from build123d import *

# Parameters (mm, degrees)
BOSS_EXTRU_1_DEPTH                              = 8
CHAMBRAGE_POUR_VIS_T_TE_CYLINDRIQUE_D           = 2.5
CHAMBRAGE_POUR_VIS_T_TE_CYLINDRIQUE_CBORE_D     = 4.5
CHAMBRAGE_POUR_VIS_T_TE_CYLINDRIQUE_CBORE_DEPTH = 6.5
CONG_1_R                                        = 0.5
ESQUISSE6_R                                     = 1.6
ENL_V_MAT_EXTRU_1_DEPTH                         = 18.49285573
ESQUISSE7_W                                     = 6
ESQUISSE7_H                                     = 2.25
ENL_V_MAT_EXTRU_2_DEPTH                         = 18.492855685
ESQUISSE8_R                                     = 5.5
ENL_V_MAT_EXTRU_3_DEPTH                         = 3


with BuildPart() as part:
    # Esquisse1 → Boss.-Extru.1 (new body)
    with BuildSketch(Plane(origin=(0, 0, 0), x_dir=(1, 0, 0), z_dir=(0, 1, 0))):
        with BuildLine():
            Line((4.582575695, 10), (-4.582575695, 10))
            ThreePointArc((-4.582575695, 10), (0, -11), (4.582575695, 10))
        make_face()
        with BuildLine():
            Line((-3.2, 0), (-3.2, 2.9))
            Line((-3.2, 2.9), (3.2, 2.9))
            Line((3.2, 2.9), (3.2, 0))
            ThreePointArc((3.2, 0), (0, -3.2), (-3.2, 0))
        make_face(mode=Mode.SUBTRACT)
    extrude(amount=BOSS_EXTRU_1_DEPTH)

    # Chambrage pour vis à tête cylindrique à 6 pans creux (ou vis CHC) M21 (through all)
    with Locations(Plane(origin=(0, 8, 0), x_dir=(1, 0, 0), z_dir=(0, 1, 0))):
        with Locations((5.656854249, 5.656854249), (5.656854249, -5.656854249), (-5.656854249, -5.656854249), (-5.656854249, 5.656854249), (0, 0)):
            CounterBoreHole(CHAMBRAGE_POUR_VIS_T_TE_CYLINDRIQUE_D / 2, CHAMBRAGE_POUR_VIS_T_TE_CYLINDRIQUE_CBORE_D / 2, CHAMBRAGE_POUR_VIS_T_TE_CYLINDRIQUE_CBORE_DEPTH)

    # Congé1
    cong_1_edges = [part.edges().sort_by_distance(p)[0] for p in [
        (0, 8, 3.2),
        (3.2, 8, -1.45),
        (0, 8, -2.9),
        (-3.2, 8, -1.45),
    ]]
    fillet(cong_1_edges, radius=CONG_1_R)

    # Esquisse6 → Enlèv. mat.-Extru.1 (cut, through all)
    with BuildSketch(Plane.XY):
        with Locations((0, 5.5)):
            Circle(ESQUISSE6_R)
    extrude(amount=-ENL_V_MAT_EXTRU_1_DEPTH, mode=Mode.SUBTRACT)

    # Esquisse7 → Enlèv. mat.-Extru.2 (cut, through all)
    with BuildSketch(Plane(origin=(0, 8, 0), x_dir=(1, 0, 0), z_dir=(0, 1, 0))):
        with Locations((0, 5.025)):
            Rectangle(ESQUISSE7_W, ESQUISSE7_H)
    extrude(amount=-ENL_V_MAT_EXTRU_2_DEPTH, mode=Mode.SUBTRACT)

    # Esquisse8 → Enlèv. mat.-Extru.3 (cut)
    with BuildSketch(Plane(origin=(0, 0, 0), x_dir=(-1, 0, 0), z_dir=(0, -1, 0))):
        Circle(ESQUISSE8_R)
    extrude(amount=-ENL_V_MAT_EXTRU_3_DEPTH, mode=Mode.SUBTRACT)


solid = part.part
Model file for the job. Use its own axes, mm. A direction names the side the tool comes from. Give positions to 0.01 mm unless a question says otherwise; leave off trailing zeros. Write each loop counter-clockwise with the first axis right and the second up, starting at its lowest first coordinate (ties: lowest second). Pieces come first, ordered by that corner, then holes. Notation, with made-up numbers: (82, -0.75) - (98, -0.75) arc R21 ccw to (98, 20.25) - close; hole circle Ø9 at (81.5, 7.25). An arc over 180 degrees is marked (long way). Answer as CSV lines item,"result".
1. Band-saw the part on D-D (y = 5.5). Write the cut outline in (x, z), and give its area (3 significant figures).
Responses:
outline,"(-4.58, -10) - (-1.6, -10) - (-1.6, -6.15) - (-3, -6.15) - (-3, -3.9) - (-1.6, -3.9) - (-1.6, -2.9) - (-3.2, -2.9) - (-3.2, 0) arc R3.2 cw to (3.2, 0) - (3.2, -2.9) - (1.6, -2.9) - (1.6, -3.9) - (3, -3.9) - (3, -6.15) - (1.6, -6.15) - (1.6, -10) - (4.58, -10) arc R11 ccw (long way) to start; hole circle Ø4.5 at (-5.66, -5.66); hole circle Ø4.5 at (-5.66, 5.66); hole circle Ø4.5 at (5.66, -5.66); hole circle Ø4.5 at (5.66, 5.66)"
area,"247 mm2"
2. Band-saw the part on B-B (z = -1.25). Write the cut outline in (x, y).
Responses:
outline,"(-10.93, 0) - (-5.36, 0) - (-5.36, 3) - (-3.2, 3) - (-3.2, 7.5) arc R0.5 ccw to (-3.7, 8) - (-10.93, 8) - close; (3.2, 3) - (5.36, 3) - (5.36, 0) - (10.93, 0) - (10.93, 8) - (3.7, 8) arc R0.5 ccw to (3.2, 7.5) - close"
3. Band-saw the part on C-C (y = 2). Write the cut outline in (x, z).
Responses:
outline,"(-4.58, -10) - (4.58, -10) arc R11 ccw (long way) to start; hole circle Ø4.5 at (-5.66, -5.66); hole circle Ø4.5 at (-5.66, 5.66); hole (-3, -6.15) - (3, -6.15) - (3, -4.61) arc R5.5 ccw (long way) to (-3, -4.61) - close; hole circle Ø4.5 at (5.66, -5.66); hole circle Ø4.5 at (5.66, 5.66)"
4. Drill centre lines: L1, parallel to X at y = 2.5, z = -7.5; L2, parallel to X at y = 1.8, z = 0; L3, parallel to Z at x = -7, y = 7.5. Where is each one in solid material? Low to high. Write a range as [from, to].
Responses:
L1,"x = [-8.05, -6.95], [-4.37, 4.37], [6.95, 8.05]"
L2,"x = [-11, -5.5], [5.5, 11]"
L3,"z = [-8.49, -7.46], [-3.85, 3.85], [7.46, 8.49]"
5. 3-axis set-ups, long thin cutter, end or side, ignore diameter. For faces 1 (the face through (0.197, 1.479, 5.496)), 2 (the face through (7, 1.5, 7)), 3 (the face through (-0.35, 3.94, -3.39)): which of +Z, -Z, +X, -X, +Y, -Y reach the whole face in a straight line?
Responses:
face 1,"-Y"
face 2,"+Y"
face 3,"-Z"
6. Two-plate mould, pull along Z, no slides. Class faces 4 (the face through (-5, 1.5, 7)), 5 (the face through (-0.35, 3.94, -8.05)), 6 (the face through (0, 3, -10)): +Z half, -Z half, draft (parallel to the pull), parting line (faces both ways), or undercut.
Responses:
face 4,"undercut"
face 5,"draft"
face 6,"-Z half"
7. Band-saw the part on A-A (x = 0). Write the cut outline in (y, z).
Responses:
outline,"(0, -10) - (3.9, -10) - (3.9, -6.15) - (0, -6.15) - close; (0, 5.5) - (3, 5.5) - (3, 3.2) - (7.5, 3.2) arc R0.5 ccw to (8, 3.7) - (8, 11) - (0, 11) - close; (3, -3.9) - (3.9, -3.9) - (3.9, -2.9) - (3, -2.9) - close; (7.1, -10) - (8, -10) - (8, -6.15) - (7.1, -6.15) - close; (7.1, -3.9) - (8, -3.9) - (8, -3.4) arc R0.5 ccw to (7.5, -2.9) - (7.1, -2.9) - close"
8. Pin check, flat tips, straight feed: pin 1 (3 mm diameter, centred on y = 1, z = 4, fed in from -X); pin 2 (1.3 mm diameter, centred on x = -6, z = 5.5, fed in from +Y); pin 3 (3.5 mm diameter, centred on x = 5.66, z = -5.66, fed in from +Y); pin 4 (5 mm diameter, centred on x = 1.5, z = 0, fed in from -Y). Stop position of each tip, or through.
Responses:
pin 1,"stops at x = -10.71"
pin 2,"passes through"
pin 3,"stops at y = 1.5"
pin 4,"stops at y = 3"
